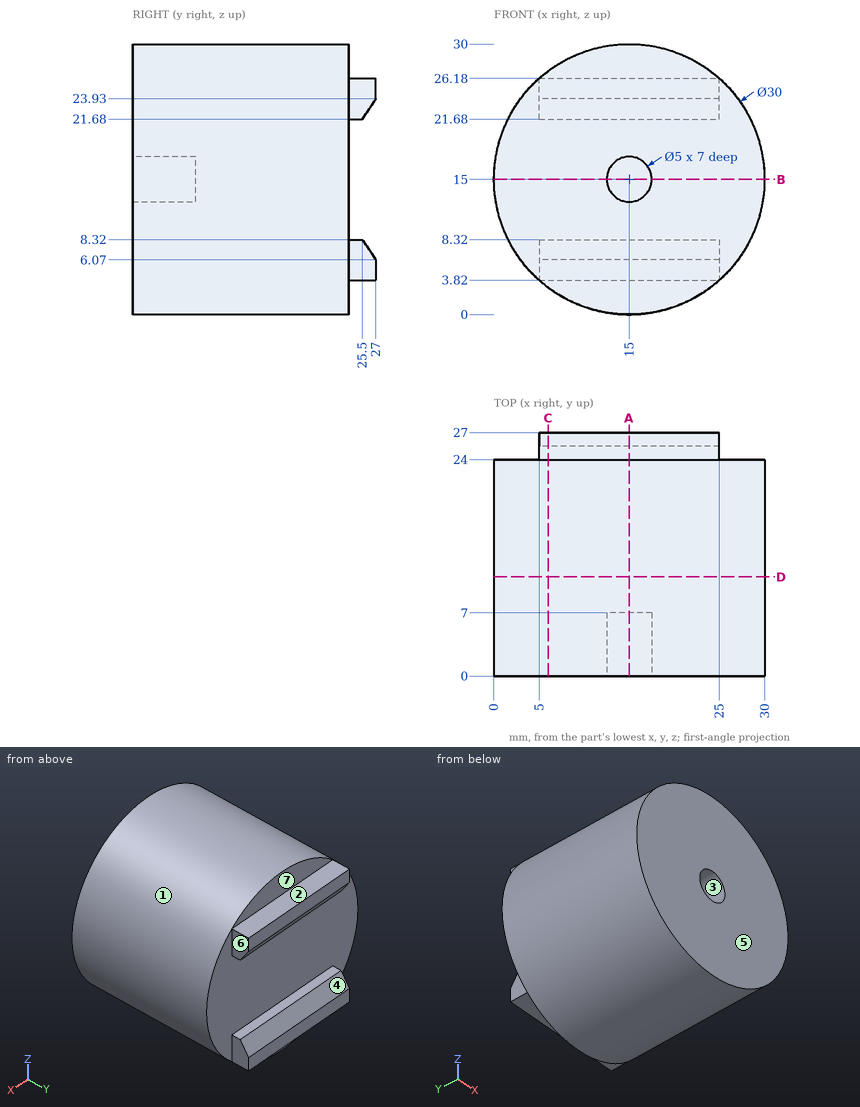
Job drawing, mm, ordinate dimensions from the low corner. One solid piece. A direction names the side the tool comes from. Give positions to 0.01 mm unless a question says otherwise; leave off trailing zeros. Order: outer loops, then holes, each group sorted by start corner. A loop starts at its lowest first (then second) coordinate and runs counter-clockwise, first axis right, second up. Notation, with made-up numbers: (-17, -8) -> (39, -8) arc R32 cw to (39, 24) -> close; hole circle Ø4 at (-4, 7). An arc over 180 degrees is marked (long way). Return JSON: item names as keys, results as strings.
Q1. Mould opens along X. For the marked faces 1, 2 and 3 say: pulls with the +X half, pulls with the -X half, needs draft (parallel to the pull), parting line crosses it, or undercut.
Working result:
{"face 1": "parting line crosses it", "face 2": "needs draft", "face 3": "undercut"}
Q2. Saw through at A-A (x = 15). Write the cut outline in (y, z), then the cut area to 3 significant figures.
Working result:
{"outline": "(0, 0) -> (24, 0) -> (24, 3.82) -> (27, 3.82) -> (27, 6.07) -> (25.5, 8.32) -> (24, 8.32) -> (24, 21.68) -> (25.5, 21.68) -> (27, 23.93) -> (27, 26.18) -> (24, 26.18) -> (24, 30) -> (0, 30) -> (0, 17.5) -> (7, 17.5) -> (7, 12.5) -> (0, 12.5) -> close", "area": "709 mm²"}
Q3. Saw through at C-C (x = 6). Write the cut outline in (y, z).
Working result:
{"outline": "(0, 3) -> (24, 3) -> (24, 3.82) -> (27, 3.82) -> (27, 6.07) -> (25.5, 8.32) -> (24, 8.32) -> (24, 21.68) -> (25.5, 21.68) -> (27, 23.93) -> (27, 26.18) -> (24, 26.18) -> (24, 27) -> (0, 27) -> close"}
Q4. Which spindle directions (+Z, -Z, +X, -X, +Y, -Y) get a long thin tool onto all of the face, cutting with end or side? Do the marked faces 4, 5, 6 and 7. Say none if no direction does.
Working result:
{"face 4": "+X, -X, +Y", "face 5": "+Z, -Z, +X, -X, -Y", "face 6": "+Z, -Z, +X, +Y", "face 7": "+Z, +X, -X, +Y"}
Q5. Saw through at B-B (z = 15). Write the cut outline in (x, y).
Working result:
{"outline": "(0, 0) -> (12.5, 0) -> (12.5, 7) -> (17.5, 7) -> (17.5, 0) -> (30, 0) -> (30, 24) -> (0, 24) -> close"}
Q6. Flat gauge pins, fed straight in: pin 1 (1.5 mm diameter, centred on y = 25, z = 7, fed in from +X); pin 2 (1.5 mm diameter, centred on x = 12, y = 26, fed in from +Z); pin 3 (4 mm diameter, centred on x = 11.5, z = 1, fed in from +Y). Where does each tip first touch, or does it go through?
Working result:
{"pin 1": "x = 25", "pin 2": "z = 26.18", "pin 3": "y = 24"}
Q7. Saw through at D-D (y = 11). Write the cut outline in (x, z), then the cut area to 3 significant figures.
Working result:
{"outline": "circle Ø30 at (15, 15)", "area": "707 mm²"}
Q8. Drill centre lines: line 1 (X direction, y = 3.25, z = 15); line 2 (Y direction, x = 12.5, z = 20.75); line 3 (X direction, y = 3.75, z = 16). Where is each one in solid material? Low to high.
Working result:
{"line 1": "0 to 12.5, 17.5 to 30", "line 2": "0 to 24", "line 3": "0.03 to 12.71, 17.29 to 29.97"}
